from build123d import *

# Parameters (mm, degrees)
SKETCH019_R     = 8
SKETCH019_R_2   = 2.5
PAD010_DEPTH    = 5
SKETCH020_R     = 7
SKETCH020_R_2   = 3.5
POCKET010_DEPTH = 0.5
SKETCH021_R     = 7
SKETCH021_R_2   = 3.5
POCKET011_DEPTH = 0.5


with BuildPart() as part:
    # Sketch019 → Pad010 (new body)
    with BuildSketch(Plane.XY):
        Circle(SKETCH019_R)
        Circle(SKETCH019_R_2, mode=Mode.SUBTRACT)
    extrude(amount=PAD010_DEPTH)

    # Sketch020 → Pocket010 (cut)
    with BuildSketch(Plane.XY.offset(5)):
        Circle(SKETCH020_R)
        Circle(SKETCH020_R_2, mode=Mode.SUBTRACT)
    extrude(amount=-POCKET010_DEPTH, mode=Mode.SUBTRACT)

    # Sketch021 → Pocket011 (cut)
    with BuildSketch(Plane.XY):
        Circle(SKETCH021_R)
        Circle(SKETCH021_R_2, mode=Mode.SUBTRACT)
    extrude(amount=POCKET011_DEPTH, mode=Mode.SUBTRACT)


solid = part.part
For this review, take the finished solid that the model builds, in its own axes (mm). A direction names the side the tool comes from. Round coordinates to 2 decimals unless told otherwise and drop trailing zeros. Order: outer loops, then holes, each group sorted by start corner. A loop starts at its lowest first (then second) coordinate and runs counter-clockwise, first axis right, second up. Notation, with made-up numbers: (57.25, 21.5) -> (67.25, 21.5) arc R25 cw to (67.25, 46.5) -> close; hole circle Ø6 at (-1, 76). An arc over 180 degrees is marked (long way). Write item = value, one per line. Start each with the question number.
1) Insertion check: pin 1 (3 mm diameter, centred on x = 6, z = 2, fed in from -Y); pin 2 (3 mm diameter, centred on x = 0, y = 0, fed in from -Z); pin 3 (2 mm diameter, centred on x = 6, z = 2, fed in from -Y) (3 decimals); pin 4 (1 mm diameter, centred on x = 6, y = 2, fed in from +Z). Each pin has a flat end and moves straight along its axis. Give the tip position at first contact, or say it passes through.
2) Take a section at A-A on x = 0. State the section outline as (y, z) points, plus the area to 3 significant figures.
3) The part is to be moulded in two halves that separate along X. For faces 4 (the face through (-1.73, -7.81, 2.46)), 5 (the face through (3, -3, 0.5)), 6 (the face through (2, -2, 0)), say which applies: +X half, -X half, draft (parallel to the pull), parting line (faces both ways), or undercut.
4) Tool access review of faces 1 (the face through (3, -3, 4.5)), 2 (the face through (4, -6, 0)), 3 (the face through (6.466, -2.681, 0.246)): name each direction out of +Z, -Z, +X, -X, +Y, -Y from which nothing blocks a thin tool from reaching the whole face with its end or side.
5) To check wall thickness, follow line 1 (Y direction, x = 0, z = 4.9); line 2 (Z direction, x = -1, y = -4.25); line 3 (Y direction, x = 0.25, z = 3.1). State the ranges of each line that lie inside material, in increasing order. Write a range as from..to.
6) Take a section at C-C on y = -3.25. State the section outline as (x, z) points, plus the area to 3 significant figures.
7) Take a section at D-D on z = 2. State the section outline as (x, y) points, plus the area to 3 significant figures.
Verdict:
q1.pin_1 = -6.61
q1.pin_2 = through
q1.pin_3 = -6.245
q1.pin_4 = 4.5
q2.outline = (-8, 0) -> (-7, 0) -> (-7, 0.5) -> (-3.5, 0.5) -> (-3.5, 0) -> (-2.5, 0) -> (-2.5, 5) -> (-3.5, 5) -> (-3.5, 4.5) -> (-7, 4.5) -> (-7, 5) -> (-8, 5) -> close; (2.5, 0) -> (3.5, 0) -> (3.5, 0.5) -> (7, 0.5) -> (7, 0) -> (8, 0) -> (8, 5) -> (7, 5) -> (7, 4.5) -> (3.5, 4.5) -> (3.5, 5) -> (2.5, 5) -> close
q2.area = 48.0 mm2
q3.face_4 = parting line
q3.face_5 = undercut
q3.face_6 = draft
q4.face_1 = +Z
q4.face_2 = -Z, +X, -X, +Y, -Y
q4.face_3 = -Z
q5.line_1 = -8..-7, -3.5..-2.5, 2.5..3.5, 7..8
q5.line_2 = 0.5..4.5
q5.line_3 = -8..-2.49, 2.49..8
q6.outline = (-7.31, 0) -> (-6.2, 0) -> (-6.2, 0.5) -> (-1.3, 0.5) -> (-1.3, 0) -> (1.3, 0) -> (1.3, 0.5) -> (6.2, 0.5) -> (6.2, 0) -> (7.31, 0) -> (7.31, 5) -> (6.2, 5) -> (6.2, 4.5) -> (1.3, 4.5) -> (1.3, 5) -> (-1.3, 5) -> (-1.3, 4.5) -> (-6.2, 4.5) -> (-6.2, 5) -> (-7.31, 5) -> close
q6.area = 63.3 mm2
q7.outline = circle Ø16 at (0, 0); hole circle Ø5 at (0, 0)
q7.area = 181 mm2
